from build123d import *

# Parameters (mm, degrees)
IZIM1_W                              = 200
IZIM1_H                              = 50
Y_KSEKLIK_EKSTR_ZYON1_DEPTH          = 8
M5_HELISARMAL_I_IN_Z_VANA_MATKAB_1_D = 5.2
KES_EKSTR_ZYON1_DEPTH                = 10
KES_EKSTR_ZYON1_DEPTH_BACK           = 10
IZIM5_R                              = 1.25
IZIM5_R_2                            = 11.5
M5_HELISARMAL_I_IN_Z_VANA_MATKAB_2_D = 5.2


with BuildPart() as part:
    # Çizim1 → Yükseklik-Ekstrüzyon1 (new body)
    with BuildSketch(Plane.XY):
        with Locations((11.855409505, 24.184782609)):
            Rectangle(IZIM1_W, IZIM1_H)
    extrude(amount=Y_KSEKLIK_EKSTR_ZYON1_DEPTH)

    # M5 Helisarmal için Zıvana matkabı1 (through all)
    with Locations(Plane(origin=(0, 0, 0), x_dir=(-1, 0, 0), z_dir=(0, 0, -1))):
        with Locations((-101.855409505, 39.184782609), (-101.855409505, 9.184782609), (78.144590495, 9.184782609), (78.144590495, 39.184782609)):
            Hole(M5_HELISARMAL_I_IN_Z_VANA_MATKAB_1_D / 2)

    # Çizim5 → Kes-Ekstrüzyon1 (cut, two sides: drawn at the far end of the back side and taken through both)
    with BuildSketch(Plane(origin=(0, 0, 0), x_dir=(-1, 0, 0), z_dir=(0, 0, -1)).offset(-KES_EKSTR_ZYON1_DEPTH_BACK)):
        with Locations((3.644590495, 39.684782609)):
            Circle(IZIM5_R)
        with Locations((3.075905377, 8.684782609)):
            Circle(IZIM5_R)
        with Locations((-27.924094623, 9.544465449)):
            Circle(IZIM5_R)
        with Locations((-27.355409505, 40.544465449)):
            Circle(IZIM5_R)
        with Locations((-11.855409505, 24.184782609)):
            Circle(IZIM5_R_2)
    extrude(amount=KES_EKSTR_ZYON1_DEPTH + KES_EKSTR_ZYON1_DEPTH_BACK, mode=Mode.SUBTRACT)

    # M5 Helisarmal için Zıvana matkabı2 (through all)
    with Locations(Plane(origin=(71.855409505, 9.184782609, 0), x_dir=(-1, 0, 0), z_dir=(0, 0, -1))):
        with Locations((0, 0), (120, 0)):
            Hole(M5_HELISARMAL_I_IN_Z_VANA_MATKAB_2_D / 2)


solid = part.part
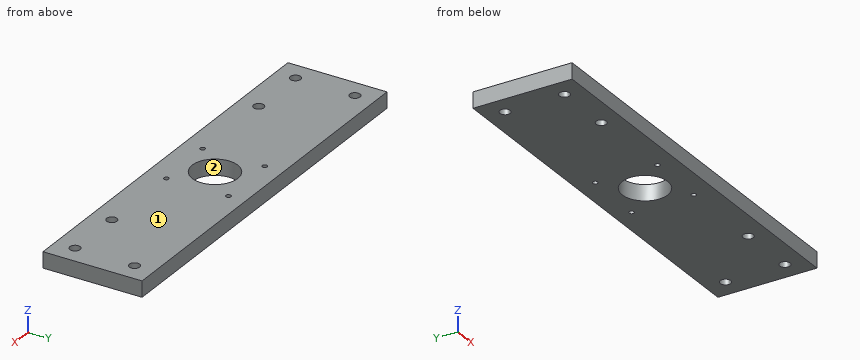
CAD build for the part. Positions are in the model's coordinates, mm. Face numbers are marked on the shaded views. Round coordinates to 2 decimals unless told otherwise and drop trailing zeros. Order: outer loops, then holes, each group sorted by start corner. A loop starts at its lowest first (then second) coordinate and runs counter-clockwise, first axis right, second up. Notation, with made-up numbers: M 18,6 L 60,6 A27 cw 60,42 Z; hole C 37.25,-6 d7. An arc over 180 degrees is marked long. Use one line per item in the form item = value.
Q1. Saw through at C-C on y = 30. Give the cut face in (x, z), then the cut area to 3 significant figures.
Recorded:
outline = M -88.14,0 L 1.93,0 L 1.93,8 L -88.14,8 Z; M 21.78,0 L 111.86,0 L 111.86,8 L 21.78,8 Z
area = 1,440 mm^2
Q2. Two-plate mould, pull along Y, no slides. Class the marked faces 1 and 2: +Y half, -Y half, draft (parallel to the pull), parting line (faces both ways), or undercut.
Recorded:
face_1 = draft
face_2 = undercut
Q3. Probe L1, parallel to X at y = 33, z = 6.5; L2, parallel to X at y = 39, z = 7.75; L3, parallel to X at y = 32, z = 7.25. List the from-to ranges inside material, lowest first.
Recorded:
L1 = -88.14 to 4.47, 19.24 to 111.86
L2 = -88.14 to -80.74, -75.55 to -4.69, -2.6 to 99.26, 104.45 to 111.86
L3 = -88.14 to 3.42, 20.29 to 111.86
Q4. Saw through at B-B on z = 5.25. State how many separate pieces and enclosed holes the cut face has, then the cut area to 3 significant figures.
Recorded:
separate_pieces = 1
enclosed_holes = 11
area = 9,440 mm^2
Q5. Saw through at A-A on y = 14.5. Give the cut face in (x, z), then the cut area to 3 significant figures.
Recorded:
outline = M -88.14,0 L 5.65,0 L 5.65,8 L -88.14,8 Z; M 18.06,0 L 111.86,0 L 111.86,8 L 18.06,8 Z
area = 1,500 mm^2
Q6. Flat gauge pin, fed straight in: P1, Ø3, axis at x = 27.92, y = 9.54, coming from the +Z side. Where does the tip first touch, or does it go through?
Recorded:
P1 = 8
